Input: part model. Units: mm. Frame: model coordinates. A direction names the side the tool comes from. Coordinates: 2 decimals unless noted, no trailing zeros. Write each loop counter-clockwise with the first axis right and the second up, starting at its lowest first coordinate (ties: lowest second). Pieces come first, ordered by that corner, then holes. Notation, with made-up numbers: (-13, -35) - (41, -35) arc R11 ccw to (41, -21) - close; hole circle Ø7 at (53, -23.75). An arc over 180 degrees is marked (long way). Use a Markdown table: item, result. Add a question column.
Q1. Section query A-A (x = -23). Return the cut outline in (y, z).
Q2. Section query C-C (z = 10). Return the cut outline in (x, y), then the cut area to 3 significant figures.
Q3. Material intervals for probe 1 along X at (y, z) = (8.5, 2); probe 2 along X at (y, z) = (3.25, 15.75); probe 3 along Y at (x, z) = (7, 16), sorted ascending. Write a range as from..to.
Q4. Pin query (flat end, axial travel): P1, Ø6.5, axis at x = -30.35, z = -15.75, coming from the +Y side; P2, Ø1.6, axis at x = -3, z = -15.5, coming from the +Y side; P3, Ø2, axis at x = -30.35, z = 15.75, coming from the +Y side. Return the tip coordinate at first contact, or that it passes through.
Q5. Section query B-B (z = 15.75). Give the number of separate pieces and of enclosed holes in the cut face, then the cut area to 3 significant figures.
Q6. Set-up query: faces 4 (the face through (23, 2.72, -21)), 5 (the face through (-29, 9.22, -15)), 6 (the face through (41, 4.76, 1)). Return all of +Z, -Z, +X, -X, +Y, -Y with unobstructed straight access to the full face (end or side cutting, diameter ignored); none if empty.
Q7. Mould query, pull axis Y, two halves, no side actions, for faces 1 (the face through (40.35, 4, 1)), 2 (the face through (-3, 9, 7.77)), 3 (the face through (37, 8.22, 11)). Classes: released by +Y, released by -Y, zero draft, split by the parting line, or undercut.
from build123d import *

# Parameters (mm, degrees)
SKETCH1_W           = 84.7
SKETCH1_H           = 44.8
BOSS_EXTRUDE1_DEPTH = 10.22
SKETCH2_W           = 24.5
SKETCH2_H           = 16.3
BOSS_EXTRUDE2_DEPTH = 2
SKETCH3_W           = 5.34
SKETCH3_H           = 11.9
SKETCH3_H_2         = 9.1
SKETCH3_H_3         = 8
SKETCH3_H_4         = 17.2
SKETCH3_H_5         = 11.1
SKETCH3_H_6         = 15.17
SKETCH3_H_7         = 17.32
SKETCH3_H_8         = 13
CUT_EXTRUDE1_DEPTH  = 2
SKETCH4_R           = 1.25
CUT_EXTRUDE2_DEPTH  = 50.443006583
SKETCH5_R           = 2
CUT_EXTRUDE3_DEPTH  = 1
SKETCH6_W           = 8.64
SKETCH6_H           = 4.92
CUT_EXTRUDE4_DEPTH  = 2
SKETCH7_W           = 5
SKETCH7_H           = 2
CUT_EXTRUDE5_DEPTH  = 2
SKETCH8_W           = 20.33
SKETCH8_H           = 3.1
SKETCH8_W_2         = 5.5
SKETCH8_H_2         = 2
CUT_EXTRUDE6_DEPTH  = 2
SKETCH9_W           = 13.9
SKETCH9_H           = 2.2
CUT_EXTRUDE7_DEPTH  = 2
CUT_EXTRUDE8_DEPTH  = 0.1


with BuildPart() as part:
    # Sketch1 → Boss-Extrude1 (new body)
    with BuildSketch(Plane(origin=(0, 0, 0), x_dir=(1, 0, 0), z_dir=(0, 1, 0))):
        Rectangle(SKETCH1_W, SKETCH1_H)
    extrude(amount=BOSS_EXTRUDE1_DEPTH)

    # Sketch2 → Boss-Extrude2 (add)
    with BuildSketch(Plane(origin=(0, 10.22, 0), x_dir=(1, 0, 0), z_dir=(0, 1, 0))):
        with Locations((-30.1, 0)):
            Rectangle(SKETCH2_W, SKETCH2_H)
    extrude(amount=BOSS_EXTRUDE2_DEPTH)

    # Sketch3 → Cut-Extrude1 (cut)
    with BuildSketch(Plane(origin=(0, 10.22, 0), x_dir=(1, 0, 0), z_dir=(0, 1, 0))):
        with Locations((-37.74, -14.1)):
            Rectangle(SKETCH3_W, SKETCH3_H)
        with Locations((-23.15, -14.1)):
            Rectangle(SKETCH3_W, SKETCH3_H)
        with Locations((-2.92, -15.5)):
            Rectangle(SKETCH3_W, SKETCH3_H_2)
        with Locations((5.22, -15.5)):
            Rectangle(SKETCH3_W, SKETCH3_H_2)
        with Locations((13.46, -15.5)):
            Rectangle(SKETCH3_W, SKETCH3_H_2)
        with Locations((21.6, -16.05)):
            Rectangle(SKETCH3_W, SKETCH3_H_3)
        with Locations((21.6, -4.95)):
            Rectangle(SKETCH3_W, SKETCH3_H_3)
        with Locations((36.88, -11.45)):
            Rectangle(SKETCH3_W, SKETCH3_H_4)
        with Locations((-2.92, -1.82)):
            Rectangle(SKETCH3_W, SKETCH3_H)
        with Locations((5.22, -1.82)):
            Rectangle(SKETCH3_W, SKETCH3_H)
        with Locations((13.46, -3.22)):
            Rectangle(SKETCH3_W, SKETCH3_H_2)
        with Locations((-2.92, 13.95)):
            Rectangle(SKETCH3_W, SKETCH3_H)
        with Locations((5.22, 14.35)):
            Rectangle(SKETCH3_W, SKETCH3_H_5)
        with Locations((13.46, 12.315)):
            Rectangle(SKETCH3_W, SKETCH3_H_6)
        with Locations((21.6, 11.24)):
            Rectangle(SKETCH3_W, SKETCH3_H_7)
        with Locations((29.24, 0.8)):
            Rectangle(SKETCH3_W, SKETCH3_H_8)
        with Locations((36.88, 11.3)):
            Rectangle(SKETCH3_W, SKETCH3_H_4)
    extrude(amount=-CUT_EXTRUDE1_DEPTH, mode=Mode.SUBTRACT)

    # Sketch4 → Cut-Extrude2 (cut, through all)
    with BuildSketch(Plane.XZ):
        with Locations(Location((-30.35, 15.75, 0), (0, 0, 270))):
            Circle(SKETCH4_R)
        with Locations(Location((31.25, 15.75, 0), (0, 0, 270))):
            Circle(SKETCH4_R)
        with Locations(Location((31.25, -15.75, 0), (0, 0, 270))):
            Circle(SKETCH4_R)
        with Locations(Location((-30.35, -15.75, 0), (0, 0, 270))):
            Circle(SKETCH4_R)
    extrude(amount=-CUT_EXTRUDE2_DEPTH, mode=Mode.SUBTRACT)

    # Sketch5 → Cut-Extrude3 (cut)
    with BuildSketch(Plane(origin=(0, 10.22, 0), x_dir=(1, 0, 0), z_dir=(0, 1, 0))):
        with Locations(Location((-30.35, 15.75, 0), (0, 0, 270))):
            Circle(SKETCH5_R)
        with Locations(Location((-30.35, -15.75, 0), (0, 0, 270))):
            Circle(SKETCH5_R)
        with Locations(Location((31.25, 15.75, 0), (0, 0, 270))):
            Circle(SKETCH5_R)
        with Locations(Location((31.25, -15.75, 0), (0, 0, 270))):
            Circle(SKETCH5_R)
    extrude(amount=-CUT_EXTRUDE3_DEPTH, mode=Mode.SUBTRACT)

    # Sketch6 → Cut-Extrude4 (cut)
    with BuildSketch(Plane.XY.offset(22.4)):
        with Locations((-11.48, 5.66)):
            Rectangle(SKETCH6_W, SKETCH6_H)
    extrude(amount=-CUT_EXTRUDE4_DEPTH, mode=Mode.SUBTRACT)

    # Sketch7 → Cut-Extrude5 (cut)
    with BuildSketch(Plane.XY.offset(22.4)):
        with Locations((23.75, 3.72)):
            Rectangle(SKETCH7_W, SKETCH7_H)
    extrude(amount=-CUT_EXTRUDE5_DEPTH, mode=Mode.SUBTRACT)

    # Sketch8 → Cut-Extrude6 (cut)
    with BuildSketch(Plane(origin=(0, 0, -22.4), x_dir=(-1, 0, 0), z_dir=(0, 0, -1))):
        with Locations((-2.885, 3.3)):
            Rectangle(SKETCH8_W, SKETCH8_H)
        with Locations((-23.2, 3.72)):
            Rectangle(SKETCH8_W_2, SKETCH8_H_2)
    extrude(amount=-CUT_EXTRUDE6_DEPTH, mode=Mode.SUBTRACT)

    # Sketch9 → Cut-Extrude7 (cut)
    with BuildSketch(Plane(origin=(42.35, 0, 0), x_dir=(0, 0, -1), z_dir=(1, 0, 0))):
        with Locations((-1.25, 3.66)):
            Rectangle(SKETCH9_W, SKETCH9_H)
    extrude(amount=-CUT_EXTRUDE7_DEPTH, mode=Mode.SUBTRACT)

    # Sketch10 → Cut-Extrude8 (cut)
    with BuildSketch(Plane(origin=(0, 12.22, 0), x_dir=(1, 0, 0), z_dir=(0, 1, 0))):
        with BuildLine():
            Line((-34.034433703, 0), (-24.634433703, 2.15))
            Line((-24.634433703, 2.15), (-25.369176186, 1.392199815))
            ThreePointArc((-25.369176186, 1.392199815), (-25.933286331, 0), (-25.369176186, -1.392199815))
            Line((-25.369176186, -1.392199815), (-24.634433703, -2.15))
            Line((-24.634433703, -2.15), (-34.034433703, 0))
        make_face()
    extrude(amount=-CUT_EXTRUDE8_DEPTH, mode=Mode.SUBTRACT)


solid = part.part
Values follow:
| question | item | result |
|---|---|---|
| 1 | outline | (0, -22.4) - (10.22, -22.4) - (10.22, -8.15) - (12.22, -8.15) - (12.22, 8.15) - (8.22, 8.15) - (8.22, 20.05) - (10.22, 20.05) - (10.22, 22.4) - (0, 22.4) - close |
| 2 | outline | (-42.35, 0) - (42.35, 0) - (42.35, 10.22) - (39.55, 10.22) - (39.55, 8.22) - (34.21, 8.22) - (34.21, 10.22) - (-20.48, 10.22) - (-20.48, 8.22) - (-25.82, 8.22) - (-25.82, 10.22) - (-35.07, 10.22) - (-35.07, 8.22) - (-40.41, 8.22) - (-40.41, 10.22) - (-42.35, 10.22) - close |
| 2 | area | 834 mm2 |
| 3 | probe 1 | -42.35..-5.59, -0.25..2.55, 7.89..10.79, 16.13..18.93, 24.27..26.57, 31.91..42.35 |
| 3 | probe 2 | -42.35..-31.6, -29.1..30, 32.5..42.35 |
| 3 | probe 3 | 0..8.22 |
| 4 | P1 | y = 10.22 |
| 4 | P2 | y = 8.22 |
| 4 | P3 | through |
| 5 | separate pieces | 3 |
| 5 | enclosed holes | 0 |
| 5 | area | 737 mm2 |
| 6 | face 4 | -Z |
| 6 | face 5 | +Y |
| 6 | face 6 | +X |
| 7 | face 1 | undercut |
| 7 | face 2 | zero draft |
| 7 | face 3 | released by +Y |
